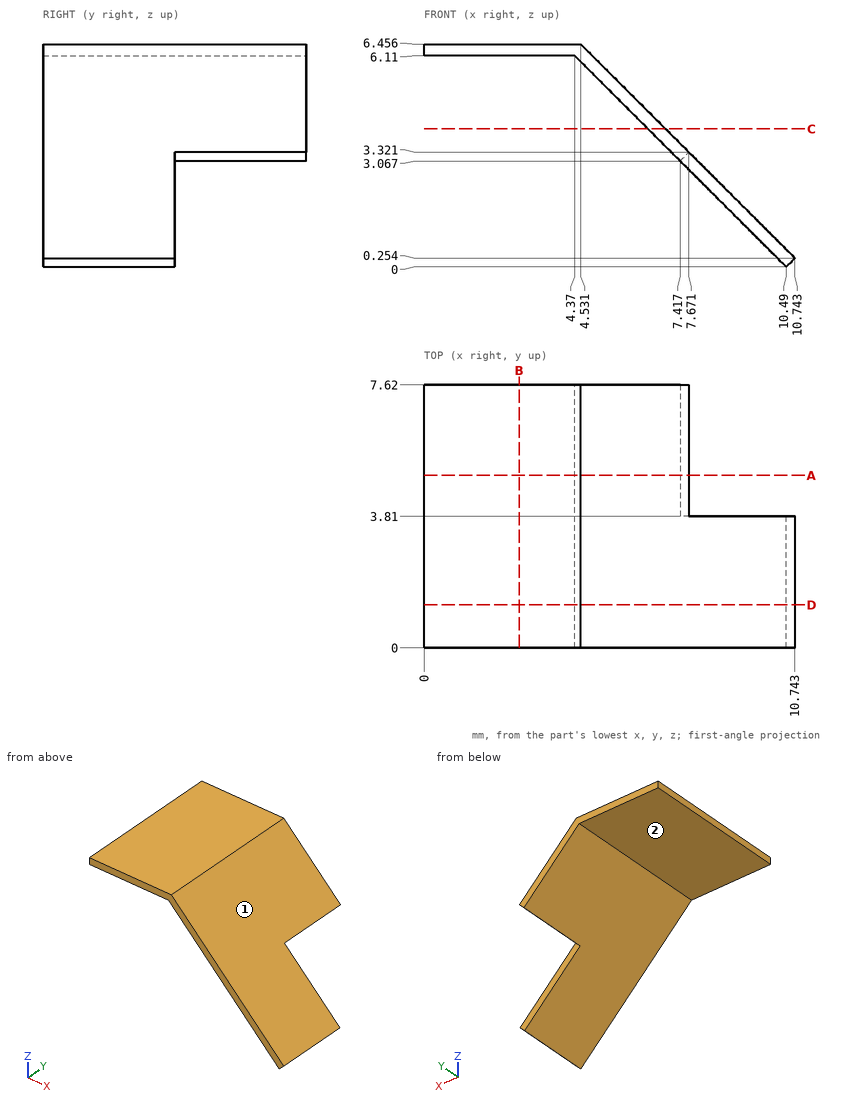
Verification items for this drawing (mm, ordinates from the low corner). A direction names the side the tool comes from. Round coordinates to 2 decimals unless told otherwise and drop trailing zeros. Order: outer loops, then holes, each group sorted by start corner. A loop starts at its lowest first (then second) coordinate and runs counter-clockwise, first axis right, second up. Notation, with made-up numbers: (-31.5, 68.5) - (-5.5, 68.5) arc R20 cw to (-5.5, 77.5) - close; hole circle Ø11 at (82.5, -25). An arc over 180 degrees is marked (long way). Use CSV: the item, a comma, the result in double quotes. Start each with the question number.
1) Thickness scan on L1, parallel to Z at x = 1.75, y = 4.75; L2, parallel to X at y = 3.75, z = 0.75 (1 decimal); L3, parallel to Z at x = 9.5, y = 2.25 (1 decimal). Record the ranges inside material, lowest first.
2) Section check B-B, the plane x = 2.75. Record the cut outline in (y, z).
3) Section check C-C, the plane z = 4. Record the cut outline in (x, y).
4) Access from +Z, -Z, +X, -X, +Y, -Y to the whole of each face (thin tool, end or side, straight path). Record for the marked faces 1 and 2.
5) Section check A-A, the plane y = 5. Record the cut outline in (x, z).
6) Go/stop test with flat-tipped pins: P1, Ø1.7, axis at x = 9.5, z = 2.5, coming from the +Y side; P2, Ø2, axis at x = 7, y = 4, coming from the +Z side; P3, Ø1.5, axis at x = 6, y = 1.5, coming from the +Z side. Record where each tip stops, or that it passes through.
7) Section check D-D, the plane y = 1.25. Record the cut outline in (x, z).
Answers:
1,L1,"z = 6.11 to 6.46"
1,L2,"x = 9.7 to 10.2"
1,L3,"z = 1 to 1.5"
2,outline,"(0, 6.11) - (7.62, 6.11) - (7.62, 6.46) - (0, 6.46) - close"
3,outline,"(6.48, 0) - (6.99, 0) - (6.99, 7.62) - (6.48, 7.62) - close"
4,face 1,"+Z, +X, +Y, -Y"
4,face 2,"-Z, -X, +Y, -Y"
5,outline,"(0, 6.11) - (4.37, 6.11) - (7.42, 3.07) - (7.67, 3.32) - (4.53, 6.46) - (0, 6.46) - close"
6,P1,"stops at y = 3.81"
6,P2,"stops at z = 4.99"
6,P3,"stops at z = 5.74"
7,outline,"(0, 6.11) - (4.37, 6.11) - (10.49, 0) - (10.74, 0.25) - (4.53, 6.46) - (0, 6.46) - close"
